Drawing for the job (mm, zero at the part's lowest x, y, z). A direction names the side the tool comes from. Coordinates: 2 decimals unless noted, no trailing zeros. Write each loop counter-clockwise with the first axis right and the second up, starting at its lowest first coordinate (ties: lowest second). Pieces come first, ordered by that corner, then holes. Notation, with made-up numbers: M 84.25,72 L 100.25,72 A27 ccw 100.25,105 Z; hole C 88,79.5 d9. An arc over 180 degrees is marked long. Use a Markdown table: item, result. Add a question column.
Q1. Slice it at A-A on x = 10.75. Write the cut outline in (y, z) (1 decimal), then the cut area to 3 significant figures.
Q2. Slice it at D-D on z = 37.5. Write the cut outline in (x, y).
Q3. Pin check, flat tips, straight feed: pin 1 Ø4 at (x, z) = (11, 20) entering from +Y (1 decimal); pin 2 Ø4 at (x, z) = (7, 6.5) entering from +Y; pin 3 Ø12 at (x, z) = (7.5, 27.5) entering from +Y. Stop position of each tip, or through.
Q4. Slice it at B-B on y = 13. Write the cut outline in (x, z) (1 decimal).
Q5. Tool access for the marked faces 1 and 2: list every direction of +Z, -Z, +X, -X, +Y, -Y with a clear straight run to the whole face (end or side of a thin tool).
Q6. Wall check: L1, parallel to Z at x = 17.25, y = 7; L2, parallel to X at y = 16.5, z = 19.5; L3, parallel to Y at x = 17, z = 24.5. Give the ranges that are in metal, low to high. Write a range as from..to.
Q7. Slice it at C-C on z = 12.5. Write the cut outline in (x, y).
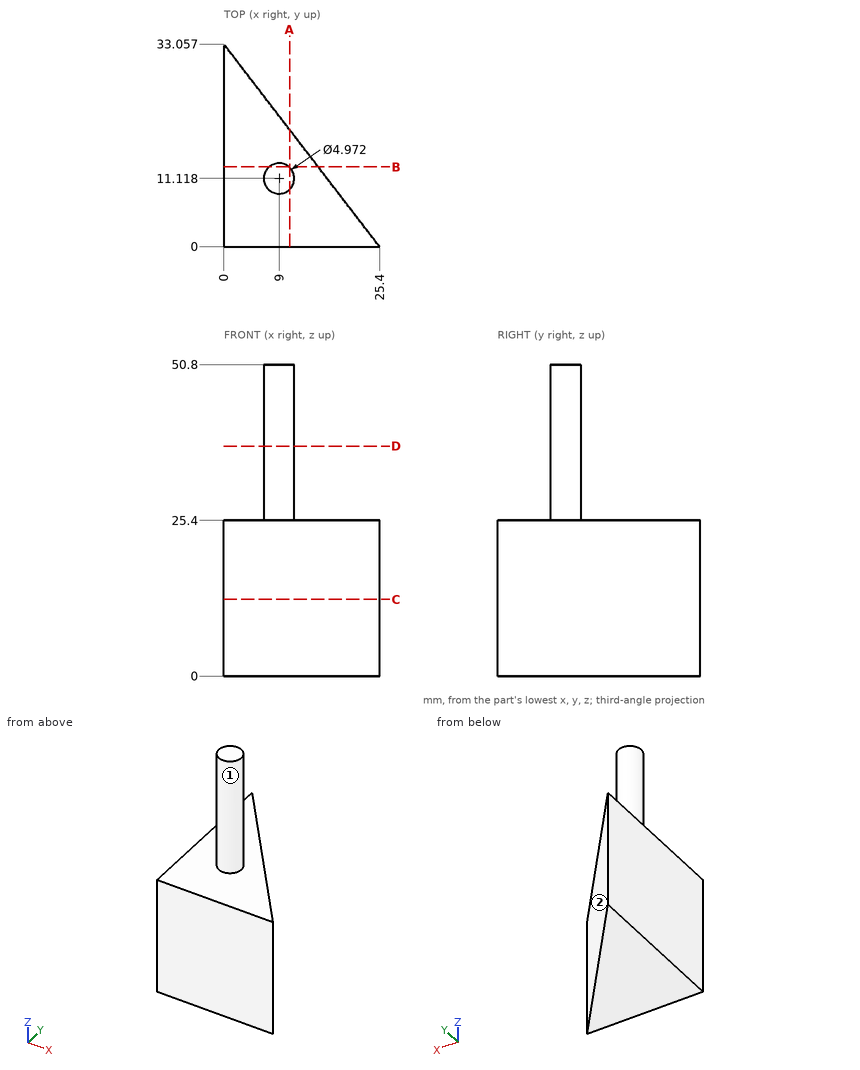
Recorded:
| question | item | result |
|---|---|---|
| 1 | outline | M 0,0 L 19.1,0 L 19.1,25.4 L 12.9,25.4 L 12.9,50.8 L 9.4,50.8 L 9.4,25.4 L 0,25.4 Z |
| 1 | area | 574 mm² |
| 2 | outline | C 9,11.12 d4.97 |
| 3 | pin 1 | y = 21.3 |
| 3 | pin 2 | y = 26.55 |
| 3 | pin 3 | y = 30.61 |
| 4 | outline | M 0,0 L 15.4,0 L 15.4,25.4 L 10.6,25.4 L 10.6,50.8 L 7.4,50.8 L 7.4,25.4 L 0,25.4 Z |
| 5 | face 1 | +Z |
| 5 | face 2 | +Z, -Z, +X, +Y |
| 6 | L1 | 0..25.4 |
| 6 | L2 | 0..12.72 |
| 6 | L3 | 0..10.93 |
| 7 | outline | M 0,0 L 25.4,0 L 0,33.06 Z |
